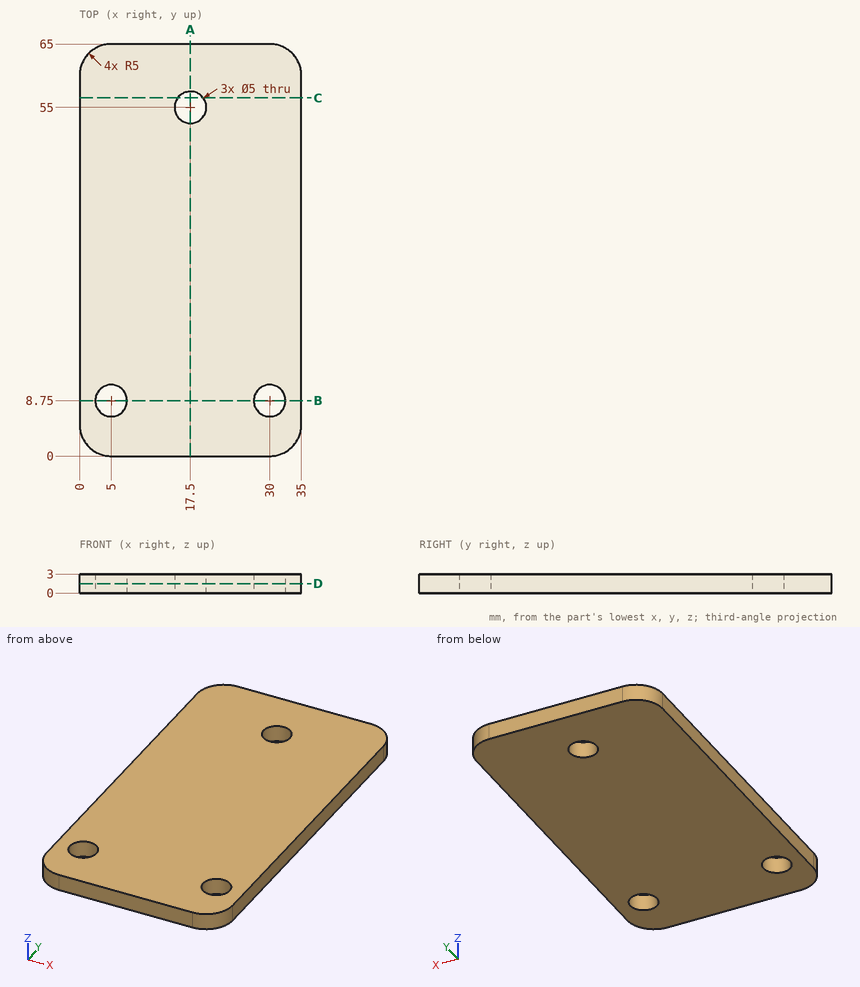
Part print with two shaded views. Sizes in mm from the minimum x, y, z corner. Coordinates: 2 decimals unless noted, no trailing zeros. Order: outer loops, then holes, each group sorted by start corner. A loop starts at its lowest first (then second) coordinate and runs counter-clockwise, first axis right, second up. Notation, with made-up numbers: (33.25, 82.25) - (54.25, 82.25) arc R11 ccw to (54.25, 93.25) - close; hole circle Ø11 at (-23, 16.5). An arc over 180 degrees is marked (long way). Answer in a Markdown table with one row per item.
1. Slice it at B-B, the plane y = 8.75. List the corners of the cut face in (x, z).
Answer:
| item | result |
|---|---|
| outline | (0, 0) - (2.5, 0) - (2.5, 3) - (0, 3) - close; (7.5, 0) - (27.5, 0) - (27.5, 3) - (7.5, 3) - close; (32.5, 0) - (35, 0) - (35, 3) - (32.5, 3) - close |
2. Slice it at D-D, the plane z = 1.5. List the corners of the cut face in (x, y), then the cut area to 3 significant figures.
Answer:
| item | result |
|---|---|
| outline | (0, 5) arc R5 ccw to (5, 0) - (30, 0) arc R5 ccw to (35, 5) - (35, 60) arc R5 ccw to (30, 65) - (5, 65) arc R5 ccw to (0, 60) - close; hole circle Ø5 at (5, 8.75); hole circle Ø5 at (17.5, 55); hole circle Ø5 at (30, 8.75) |
| area | 2,190 mm² |
3. Drill centre lines: L1, parallel to Y at x = 17.5, z = 1.6; L2, parallel to Y at x = 5, z = 1.25; L3, parallel to X at y = 9, z = 0.4. Where is each one in solid material? Low to high. Write a range as from..to.
Answer:
| item | result |
|---|---|
| L1 | 0..52.5, 57.5..65 |
| L2 | 0..6.25, 11.25..65 |
| L3 | 0..2.51, 7.49..27.51, 32.49..35 |
4. Slice it at A-A, the plane x = 17.5. List the corners of the cut face in (y, z).
Answer:
| item | result |
|---|---|
| outline | (0, 0) - (52.5, 0) - (52.5, 3) - (0, 3) - close; (57.5, 0) - (65, 0) - (65, 3) - (57.5, 3) - close |
5. Flat gauge pin, fed straight in: P1, Ø4, axis at x = 30, y = 8.75, coming from the +Z side. Where does the tip first touch, or does it go through?
Answer:
| item | result |
|---|---|
| P1 | through |
6. Slice it at C-C, the plane y = 56.5. List the corners of the cut face in (x, z).
Answer:
| item | result |
|---|---|
| outline | (0, 0) - (15.5, 0) - (15.5, 3) - (0, 3) - close; (19.5, 0) - (35, 0) - (35, 3) - (19.5, 3) - close |
